from build123d import *

# Parameters (mm, degrees)
F0_W      = 1800
F0_H      = 450
F1_DEPTH  = 10
F2_W      = 40
F2_H      = 450
F3_DEPTH  = 40
F4_W      = 40
F4_H      = 450
F5_DEPTH  = 40
F6_W      = 40
F6_H      = 370
F7_DEPTH  = 40
F8_W      = 1720
F8_H      = 40
F9_DEPTH  = 40
F10_W     = 1720
F10_H     = 40
F11_DEPTH = 40
F12_W     = 40
F12_H     = 40
F13_DEPTH = 1095
F14_W     = 40
F14_H     = 40
F15_DEPTH = 1095
F16_W     = 40
F16_H     = 40
F17_DEPTH = 1095
F18_W     = 40
F18_H     = 40
F19_DEPTH = 310
F20_W     = 40
F20_H     = 40
F21_DEPTH = 310
F22_W     = 40
F22_H     = 40
F23_DEPTH = 310


with BuildPart() as f1:
    # F0 (on Top) → F1 (new body)
    with BuildSketch(Plane.XY):
        Rectangle(F0_W, F0_H)
    extrude(amount=F1_DEPTH)

    # F2 (on face) → F3 (join)
    with BuildSketch(Plane.XY.offset(10)):
        with Locations((-880, 0)):
            Rectangle(F2_W, F2_H)
    extrude(amount=F3_DEPTH)

    # F4 (on face) → F5 (join)
    with BuildSketch(Plane.XY.offset(10)):
        with Locations((880, 0)):
            Rectangle(F4_W, F4_H)
    extrude(amount=F5_DEPTH)

    # F6 (on face) → F7 (join)
    with BuildSketch(Plane.XY.offset(10)):
        Rectangle(F6_W, F6_H)
    extrude(amount=F7_DEPTH)

    # F8 (on face) → F9 (join)
    with BuildSketch(Plane.XY.offset(10)):
        with Locations((0, -205)):
            Rectangle(F8_W, F8_H)
    extrude(amount=F9_DEPTH)

    # F10 (on face) → F11 (join)
    with BuildSketch(Plane.XY.offset(10)):
        with Locations((0, 205)):
            Rectangle(F10_W, F10_H)
    extrude(amount=F11_DEPTH)

    # F12 (on face) → F13 (join)
    with BuildSketch(Plane.XY.offset(50)):
        with Locations((-880, -205)):
            Rectangle(F12_W, F12_H)
    extrude(amount=F13_DEPTH)

    # F14 (on face) → F15 (join)
    with BuildSketch(Plane.XY.offset(50)):
        with Locations((0, -205)):
            Rectangle(F14_W, F14_H)
    extrude(amount=F15_DEPTH)

    # F16 (on face) → F17 (join)
    with BuildSketch(Plane.XY.offset(50)):
        with Locations((880, -205)):
            Rectangle(F16_W, F16_H)
    extrude(amount=F17_DEPTH)

    # F18 (on face) → F19 (join)
    with BuildSketch(Plane.XY.offset(50)):
        with Locations((-880, 205)):
            Rectangle(F18_W, F18_H)
    extrude(amount=F19_DEPTH)

    # F20 (on face) → F21 (join)
    with BuildSketch(Plane.XY.offset(50)):
        with Locations((0, 205)):
            Rectangle(F20_W, F20_H)
    extrude(amount=F21_DEPTH)

    # F22 (on face) → F23 (join)
    with BuildSketch(Plane.XY.offset(50)):
        with Locations((880, 205)):
            Rectangle(F22_W, F22_H)
    extrude(amount=F23_DEPTH)


solid = f1.part
Input: part model. Units: mm. Frame: model coordinates. A direction names the side the tool comes from. Round coordinates to 2 decimals unless told otherwise and drop trailing zeros. Loops run counter-clockwise (first coordinate to the right, second up) from the corner with the lowest first, then second, coordinate; pieces in that order, holes last. Notation, with made-up numbers: (-30, -35.75) -> (-24, -35.75) arc R19 cw to (-24, -18.75) -> close; hole circle Ø3 at (25, 70). An arc over 180 degrees is marked (long way). Answer as a JSON object with one key per item and string values. Group by question number.
1) Section query A-A on z = 246. Output: boundary loops of the cut face in (x, y).
2) Section query C-C on x = 676. Output: boundary loops of the cut face in (y, z), plus the area to 3 significant figures.
3) Section query B-B on z = 936. Output: boundary loops of the cut face in (x, y), plus the area to 3 significant figures.
4) Reachability of faces 4 (the flat face through (-900, -201, 358)), 5 (the flat face through (-880, -185, 590)), 6 (the flat face through (860, 205, 203)), 7 (the flat face through (20, -3, 30)) from +Z, -Z, +X, -X, +Y, -Y: full face, straight path, thin tool, end or side. Return the list, or none.
5) Pin query (flat end, axial travel): pin 1 (12 mm diameter, centred on x = 6, y = 57, fed in from +Z); pin 2 (4 mm diameter, centred on x = 503, y = -148, fed in from +Z); pin 3 (20 mm diameter, centred on x = -875.5, z = 462, fed in from +Y). Return the tip coordinate at first contact, or that it passes through.
6) Draft query along Y for faces 1 (the flat face through (0, -185, 590)), 2 (the flat face through (434, -205, 50)), 3 (the flat face through (-4, 225, 99)). Return one class per face: +Y half, -Y half, draft (parallel to the pull), parting line (faces both ways), or undercut.
7) Section query D-D on y = 65. Output: boundary loops of the cut face in (x, z), plus the area to 3 significant figures.
8) Ray query, L1, parallel to X at y = -188, z = 884.5; L2, parallel to Z at x = -309.5, y = 60; L3, parallel to Z at x = -3.5, y = 105. Return the intervals inside material, ascending.
Reply:
{
 "1": {"outline": "(-900, -225) -> (-860, -225) -> (-860, -185) -> (-900, -185) -> close; (-900, 185) -> (-860, 185) -> (-860, 225) -> (-900, 225) -> close; (-20, -225) -> (20, -225) -> (20, -185) -> (-20, -185) -> close; (-20, 185) -> (20, 185) -> (20, 225) -> (-20, 225) -> close; (860, -225) -> (900, -225) -> (900, -185) -> (860, -185) -> close; (860, 185) -> (900, 185) -> (900, 225) -> (860, 225) -> close"},
 "2": {"outline": "(-225, 0) -> (225, 0) -> (225, 50) -> (185, 50) -> (185, 10) -> (-185, 10) -> (-185, 50) -> (-225, 50) -> close", "area": "7,700 mm2"},
 "3": {"outline": "(-900, -225) -> (-860, -225) -> (-860, -185) -> (-900, -185) -> close; (-20, -225) -> (20, -225) -> (20, -185) -> (-20, -185) -> close; (860, -225) -> (900, -225) -> (900, -185) -> (860, -185) -> close", "area": "4,800 mm2"},
 "4": {"face 4": "+Z, -Z, -X, +Y, -Y", "face 5": "+Z, +X, -X", "face 6": "+Z, +Y, -Y", "face 7": "+Z"},
 "5": {"pin 1": "stops at z = 50", "pin 2": "stops at z = 10", "pin 3": "stops at y = -185"},
 "6": {"face 1": "undercut", "face 2": "draft", "face 3": "+Y half"},
 "7": {"outline": "(-900, 0) -> (900, 0) -> (900, 50) -> (860, 50) -> (860, 10) -> (20, 10) -> (20, 50) -> (-20, 50) -> (-20, 10) -> (-860, 10) -> (-860, 50) -> (-900, 50) -> close", "area": "22,800 mm2"},
 "8": {"L1": "x = -900 to -860, -20 to 20, 860 to 900", "L2": "z = 0 to 10", "L3": "z = 0 to 50"}
}
